```python
from build123d import *

# Parameters (mm, degrees)
SKETCH1_R               = 40
SKETCH1_R_2             = 31.5
BOSS_EXTRUDE1_DEPTH     = 6
CUT_EXTRUDE1_REACH      = 91.644
CUT_EXTRUDE1_END_RADIUS = 31.5
SKETCH2_R               = 1.25
CIRPATTERN1_COUNT       = 4


with BuildPart() as part:
    # Sketch1 → Boss-Extrude1 (new body)
    with BuildSketch(Plane.XY):
        Circle(SKETCH1_R)
        Circle(SKETCH1_R_2, mode=Mode.SUBTRACT)
    extrude(amount=BOSS_EXTRUDE1_DEPTH)

    # Cut-Extrude1: up to this cylinder (the profile starts outside it)
    cut_extrude1_end = Plane(origin=(0, 0, 3), z_dir=(0, 0, -1)) * Cylinder(CUT_EXTRUDE1_END_RADIUS, 247.288, mode=Mode.PRIVATE)
    # Sketch2 → Cut-Extrude1 (cut, up to the surface)
    with BuildSketch(Plane(origin=(0, 40, 0), x_dir=(1, 0, 0), z_dir=(0, 1, 0)), mode=Mode.PRIVATE) as cut_extrude1_sk1:
        with Locations(Location((0, -3, 0), (0, 0, 270))):
            Circle(SKETCH2_R)
    cut_extrude1_tool1 = extrude(cut_extrude1_sk1.sketch, amount=-CUT_EXTRUDE1_REACH, mode=Mode.PRIVATE) - cut_extrude1_end
    cut_extrude1 = cut_extrude1_tool1.solids().sort_by_distance((0, 40, 3))[0]
    add(cut_extrude1, mode=Mode.SUBTRACT)

    # CirPattern1: Cut-Extrude1 ×4 about axis
    cirpattern1_axis = Axis((0, 0, 6), (0, 0, -1))
    for i in range(1, CIRPATTERN1_COUNT):
        add(cut_extrude1.rotate(cirpattern1_axis, i * 360 / CIRPATTERN1_COUNT), mode=Mode.SUBTRACT)


solid = part.part
```
The listing builds one solid part. Answer for the finished solid, in the listing's coordinates (mm). Coordinates: 2 decimals unless noted, no trailing zeros. Loops run counter-clockwise (first coordinate to the right, second up) from the corner with the lowest first, then second, coordinate; pieces in that order, holes last. Notation, with made-up numbers: (26.25, 20.25) -> (72.25, 20.25) arc R34 cw to (72.25, 53.25) -> close; hole circle Ø2 at (6.5, 7.25). An arc over 180 degrees is marked (long way). Return JSON: item names as keys, results as strings. Group by question number.
(1) Find the intervals of material crossed by probe 1 along Y at (x, z) = (-34.5, 3); probe 2 along X at (y, z) = (16, 1.25); probe 3 along X at (y, z) = (-2.5, 2), in increasing order. Write a range as from..to.
(2) A cutting plane is placed at D-D on x = 23. Write down the section's boundary in (y, z), and give its area (3 significant figures).
(3) Determine the mould class of faces 1 (the cylindrical face through (-0.38, -35.8, 4.19)), 2 (the cylindrical face through (-35.8, 0.38, 4.19)), 3 (the cylindrical face through (-8.67, -39.05, 2.96)) for opening direction Y: released by +Y, released by -Y, zero draft, split by the parting line, or undercut.
(4) A cutting plane is placed at C-C on z = 3. Write down the section's boundary in (x, y), and give its area (3 significant figures).
(5) A cutting plane is placed at A-A on x = 0. Write down the section's boundary in (y, z).
(6) A cutting plane is placed at B-B on y = -25.5. Write down the section's boundary in (x, z), and give its area (3 significant figures).
(7) Given pin 1 Ø1.5 at (x, z) = (31, 4) entering from +Y; pin 2 Ø1 at (y, z) = (-25.5, 1.5) entering from -X (3 decimals); pin 3 Ø2 at (x, z) = (7.5, 3) entering from +Y, each flat-ended and moving along its own axis, determine where each tip first touches the part or whether it passes through.
The answers:
{
 "1": {"probe 1": "y = -20.24..-1.25, 1.25..20.24", "probe 2": "x = -36.66..-27.13, 27.13..36.66", "probe 3": "x = -39.92..-31.4, 31.4..39.92"},
 "2": {"outline": "(-32.73, 0) -> (-21.52, 0) -> (-21.52, 6) -> (-32.73, 6) -> close; (21.52, 0) -> (32.73, 0) -> (32.73, 6) -> (21.52, 6) -> close", "area": "134 mm^2"},
 "3": {"face 1": "zero draft", "face 2": "undercut", "face 3": "split by the parting line"},
 "4": {"outline": "(-39.98, -1.25) arc R40 ccw to (-1.25, -39.98) -> (-1.25, -31.48) arc R31.5 cw to (-31.48, -1.25) -> close; (-39.98, 1.25) -> (-31.48, 1.25) arc R31.5 cw to (-1.25, 31.48) -> (-1.25, 39.98) arc R40 ccw to start; (1.25, -39.98) arc R40 ccw to (39.98, -1.25) -> (31.48, -1.25) arc R31.5 cw to (1.25, -31.48) -> close; (1.25, 31.48) arc R31.5 cw to (31.48, 1.25) -> (39.98, 1.25) arc R40 ccw to (1.25, 39.98) -> close", "area": "1,820 mm^2"},
 "5": {"outline": "(-40, 0) -> (-31.5, 0) -> (-31.5, 1.75) -> (-40, 1.75) -> close; (-40, 4.25) -> (-31.5, 4.25) -> (-31.5, 6) -> (-40, 6) -> close; (31.5, 0) -> (40, 0) -> (40, 1.75) -> (31.5, 1.75) -> close; (31.5, 4.25) -> (40, 4.25) -> (40, 6) -> (31.5, 6) -> close"},
 "6": {"outline": "(-30.82, 0) -> (-18.49, 0) -> (-18.49, 6) -> (-30.82, 6) -> close; (18.49, 0) -> (30.82, 0) -> (30.82, 6) -> (18.49, 6) -> close", "area": "148 mm^2"},
 "7": {"pin 1": "stops at y = 26.17", "pin 2": "stops at x = -31.225", "pin 3": "stops at y = 39.47"}
}
